from build123d import *

# Parameters (mm, degrees)
SKETCH1_R           = 45
BOSS_EXTRUDE1_DEPTH = 2.8
SKETCH3_R           = 5
BOSS_EXTRUDE2_DEPTH = 10
SKETCH3_2_R         = 5
BOSS_EXTRUDE3_DEPTH = 15


with BuildPart() as part:
    # Sketch1 → Boss-Extrude1 (new body, symmetric)
    with BuildSketch(Plane(origin=(0, 0, 0), x_dir=(1, 0, 0), z_dir=(0, 1, 0))):
        Circle(SKETCH1_R)
    extrude(amount=BOSS_EXTRUDE1_DEPTH, both=True)

    # Sketch3 → Boss-Extrude2 (add)
    with BuildSketch(Plane(origin=(0, 2.8, 0), x_dir=(1, 0, 0), z_dir=(0, 1, 0))):
        Circle(SKETCH3_R)
    extrude(amount=BOSS_EXTRUDE2_DEPTH)

    # Sketch3_2 → Boss-Extrude3 (add)
    with BuildSketch(Plane(origin=(0, 2.8, 0), x_dir=(1, 0, 0), z_dir=(0, 1, 0))):
        Circle(SKETCH3_2_R)
    extrude(amount=-BOSS_EXTRUDE3_DEPTH)


solid = part.part
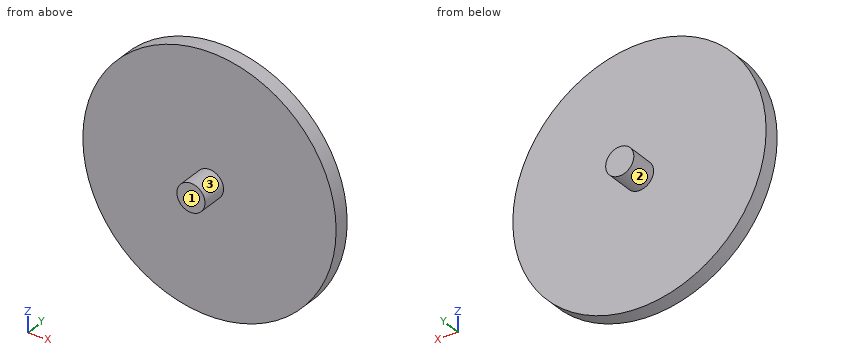
Work out the finished part from the listing and answer in its coordinate system (mm). Face numbers are marked on the shaded views. A direction names the side the tool comes from. Give positions to 0.01 mm unless a question says otherwise; leave off trailing zeros. Loops run counter-clockwise (first coordinate to the right, second up) from the corner with the lowest first, then second, coordinate; pieces in that order, holes last. Notation, with made-up numbers: M -28,28.5 L 31,28.5 A20 ccw 31,46.5 Z; hole C -8,-37.5 d6. An arc over 180 degrees is marked long. Use CSV: the item, a comma, the result in double quotes.
1) Given P1, Ø4, axis at x = 17, y = 4.5, coming from the -Z side; P2, Ø12, axis at y = -3.5, z = 30, coming from the -X side; P3, Ø1.5, axis at x = -28.5, z = 25, coming from the +Y side, each flat-ended and moving along its own axis, determine where each tip first touches the part or whether it passes through.
Answer:
P1,"z = -42.08"
P2,"x = -38.04"
P3,"y = 2.8"
2) Find section A-A on x = 0. Write down the section's boundary in (y, z).
Answer:
outline,"M -12.2,-5 L -2.8,-5 L -2.8,-45 L 2.8,-45 L 2.8,-5 L 12.8,-5 L 12.8,5 L 2.8,5 L 2.8,45 L -2.8,45 L -2.8,5 L -12.2,5 Z"
3) Find section C-C on y = -0.5. Write down the section's boundary in (x, z), plus the area to 3 significant figures.
Answer:
outline,"C 0,0 d90"
area,"6,360 mm^2"
4) Consider L1, parallel to Y at x = 37, z = -6; L2, parallel to X at y = 0.5, z = 1; L3, parallel to X at y = 4, z = -0.5. Determine where each line is inside the solid, lowest interval first.
Answer:
L1,"-2.8 to 2.8"
L2,"-44.99 to 44.99"
L3,"-4.97 to 4.97"
5) Find section B-B on z = 0. Write down the section's boundary in (x, y).
Answer:
outline,"M -45,-2.8 L -5,-2.8 L -5,-12.2 L 5,-12.2 L 5,-2.8 L 45,-2.8 L 45,2.8 L 5,2.8 L 5,12.8 L -5,12.8 L -5,2.8 L -45,2.8 Z"
6) Which of the six approach directions +Z, -Z, +X, -X, +Y, -Y give full straight-line access (tool end or side, diameter ignored) to the marked faces 1, 2 and 3?
Answer:
face 1,"+Z, -Z, +X, -X, -Y"
face 2,"+Y"
face 3,"-Y"
7) Find section D-D on y = -7.75. Write down the section's boundary in (x, z), plus the area to 3 significant figures.
Answer:
outline,"C 0,0 d10"
area,"78.5 mm^2"
